The listing builds one solid part. Answer for the finished solid, in the listing's coordinates (mm). Face numbers are marked on the shaded views. A direction names the side the tool comes from. Give positions to 0.01 mm unless a question says otherwise; leave off trailing zeros. Order: outer loops, then holes, each group sorted by start corner. A loop starts at its lowest first (then second) coordinate and runs counter-clockwise, first axis right, second up. Notation, with made-up numbers: (34.25, 56) - (68.25, 56) arc R18 cw to (68.25, 87) - close; hole circle Ø8 at (-5, 69). An arc over 180 degrees is marked (long way). Answer as a JSON object with one key per item and string values. Group by question number.
Q1. A cutting plane is placed at B-B, the plane y = -4.5. Give the vertices of the cut face in (x, z), and give its area (3 significant figures).
Q2. A cutting plane is placed at D-D, the plane y = -26. Give the vertices of the cut face in (x, z).
Q3. A cutting plane is placed at C-C, the plane x = 9.7. Give the vertices of the cut face in (y, z), and give its area (3 significant figures).
Q4. For the marked faces 4, 5, 6, 7 and 8, determine the directions among +Z, -Z, +X, -X, +Y, -Y from which every point of the face is accessible in a straight line to the end or side of a thin tool.
Q5. Consider line 1 (Z direction, x = 9.7, y = -10.35); line 2 (Y direction, x = -21, z = -1.25); line 3 (X direction, y = -25, z = 4.25). Determine where each line is inside the solid, lowest interval first.
Q6. The mould has two halves that part along Y. Classify the marked faces 1, 2 and 3: released by +Y, released by -Y, zero draft, split by the parting line, or undercut.
Q7. A cutting plane is placed at A-A, the plane x = -25.2. Give the vertices of the cut face in (y, z).
Q8. Given pin 1 (4 mm diameter, centred on x = -6.5, z = -2, fed in from +Y); pin 2 (4 mm diameter, centred on y = -21, z = 4.5, fed in from -X); pin 3 (6.5 mm diameter, centred on y = -7.5, z = 1.5, fed in from +X), each flat-ended and moving along its own axis, determine where each tip first touches the part or whether it passes through.
from build123d import *

# Parameters (mm, degrees)
BOSS_EXTRU_1_DEPTH            = 6.5
BOSS_EXTRU_1_DEPTH_BACK       = 6.5
ENL_V_MAT_EXTRU_1_DEPTH       = 2.8
ESQUISSE3_R                   = 6
BOSS_EXTRU_2_DEPTH            = 3.9
BOSS_EXTRU_3_DEPTH            = 3.8
BOSS_EXTRU_4_DEPTH            = 2
DIAM_TRE_DU_PER_AGE_4_0_4_1_D = 4
DIAM_TRE_DU_PER_AGE_4_0_4_2_D = 4
ESQUISSE10_W                  = 7
ESQUISSE10_H                  = 5
BOSS_EXTRU_5_DEPTH            = 7
D_POUILLE1_ANGLE              = 5
ESQUISSE11_W                  = 2
ESQUISSE11_H                  = 2.5
ENL_V_MAT_EXTRU_2_DEPTH       = 22.8
ENL_V_MAT_EXTRU_3_REACH       = 23.8
ESQUISSE12_W                  = 2
ESQUISSE12_H                  = 2.5


with BuildPart() as part:
    # Esquisse1 → Boss.-Extru.1 (new body, two sides)
    with BuildSketch(Plane.XY) as boss_extru_1_sk:
        Polygon((-22.5, -11.2), (-22.5, -31.2), (7, -31.2), (7, -11.2), (12, -11.2), (12, -9.4), (7, -9.4), (7, -3.7), (-22.5, -3.7), (-22.5, -9.4), (-27.5, -9.4), (-27.5, -11.2), align=None)
    extrude(amount=BOSS_EXTRU_1_DEPTH)
    extrude(boss_extru_1_sk.sketch, amount=-BOSS_EXTRU_1_DEPTH_BACK)

    # Esquisse2 → Enl_v. mat.-Extru.1 (cut)
    with BuildSketch(Plane(origin=(0, -3.7, 0), x_dir=(1, 0, 0), z_dir=(0, 1, 0))):
        Polygon((-5.5, 6.5), (-5.5, 5.5), (-21.1, 5.5), (-21.1, -5.5), (-5.5, -5.5), (-5.5, -6.5), (-22.5, -6.5), (-22.5, 6.5), align=None)
    extrude(amount=-ENL_V_MAT_EXTRU_1_DEPTH, mode=Mode.SUBTRACT)

    # Esquisse3 → Boss.-Extru.2 (add)
    with BuildSketch(Plane(origin=(0, -3.7, 0), x_dir=(1, 0, 0), z_dir=(0, 1, 0))):
        Circle(ESQUISSE3_R)
    extrude(amount=BOSS_EXTRU_2_DEPTH)

    # Esquisse4 → Boss.-Extru.3 (add)
    with BuildSketch(Plane(origin=(0, 0.2, 0), x_dir=(1, 0, 0), z_dir=(0, 1, 0))):
        Polygon((0.332133069, 2.629103958), (0, 3), (-0.332133069, 2.629103958), (-0.746069661, 2.905749483), (-0.975530065, 2.463907688), (-1.445261022, 2.62892004), (-1.557630919, 2.143895035), (-2.053641318, 2.186905882), (-2.041860093, 1.689173573), (-2.532983777, 1.607480385), (-2.397791689, 1.128315123), (-2.853169549, 0.927050983), (-2.603061214, 0.496560484), (-2.994080185, 0.188371559), (-2.64477083, -0.166394877), (-2.946861752, -0.562143944), (-2.520299768, -0.818895035), (-2.714481157, -1.277337875), (-2.237469003, -1.419941007), (-2.311539728, -1.912271969), (-1.814049831, -1.931766863), (-1.763355757, -2.427050983), (-1.276647236, -2.322212702), (-1.104373658, -2.789329458), (-0.659028201, -2.566745377), (-0.375999701, -2.976344104), (0, -2.65), (0.375999701, -2.976344104), (0.659028201, -2.566745377), (1.104373658, -2.789329458), (1.276647236, -2.322212702), (1.763355757, -2.427050983), (1.814049831, -1.931766863), (2.311539728, -1.912271969), (2.237469003, -1.419941007), (2.714481157, -1.277337875), (2.520299768, -0.818895035), (2.946861752, -0.562143944), (2.64477083, -0.166394877), (2.994080185, 0.188371559), (2.603061214, 0.496560484), (2.853169549, 0.927050983), (2.397791689, 1.128315123), (2.532983777, 1.607480385), (2.041860093, 1.689173573), (2.053641318, 2.186905882), (1.557630919, 2.143895035), (1.445261022, 2.62892004), (0.975530065, 2.463907688), (0.746069661, 2.905749483), align=None)
    extrude(amount=BOSS_EXTRU_3_DEPTH)

    # Esquisse5 → Boss.-Extru.4 (add)
    with BuildSketch(Plane(origin=(0, -3.7, 0), x_dir=(1, 0, 0), z_dir=(0, 1, 0))):
        with BuildLine():
            Line((-9.848350116, 4.9), (0, 4.9))
            Line((0, 4.9), (0, -4.9))
            Line((0, -4.9), (-9.848350116, -4.9))
            ThreePointArc((-9.848350116, -4.9), (-11, 0), (-9.848350116, 4.9))
        make_face()
    extrude(amount=BOSS_EXTRU_4_DEPTH)

    # Diam_tre du per_age _4.0 _4_1 (through all)
    with Locations(Plane(origin=(0, -9.4, 0), x_dir=(1, 0, 0), z_dir=(0, 1, 0))):
        with Locations((-25.2, 0)):
            Hole(DIAM_TRE_DU_PER_AGE_4_0_4_1_D / 2)

    # Diam_tre du per_age _4.0 _4_2 (through all)
    with Locations(Plane(origin=(0, -9.4, 0), x_dir=(1, 0, 0), z_dir=(0, 1, 0))):
        with Locations((9.7, 0)):
            Hole(DIAM_TRE_DU_PER_AGE_4_0_4_2_D / 2)

    # Esquisse10 → Boss.-Extru.5 (add)
    with BuildSketch(Plane(origin=(7, 0, 0), x_dir=(0, 0, -1), z_dir=(1, 0, 0))):
        with Locations((0, -24.7)):
            Rectangle(ESQUISSE10_W, ESQUISSE10_H)
    extrude(amount=BOSS_EXTRU_5_DEPTH)

    # D_pouille1
    d_pouille1_faces = [part.faces().sort_by_distance(p)[0] for p in [
        (10.5, -27.2, 0),
        (10.5, -24.7, -3.5),
        (10.5, -22.2, 0),
        (10.5, -24.7, 3.5),
    ]]
    draft(d_pouille1_faces, Plane(origin=(7, -11.2, -6.5), x_dir=(0, 1, 0), z_dir=(1, 0, 0)), D_POUILLE1_ANGLE)

    # Esquisse11 → Enl_v. mat.-Extru.2 (cut, through all)
    with BuildSketch(Plane(origin=(0, -9.4, 0), x_dir=(1, 0, 0), z_dir=(0, 1, 0))):
        with Locations((-26.5, 0)):
            Rectangle(ESQUISSE11_W, ESQUISSE11_H)
    extrude(amount=-ENL_V_MAT_EXTRU_2_DEPTH, mode=Mode.SUBTRACT)

    # Esquisse12 → Enl_v. mat.-Extru.3 (cut, up to next)
    with BuildSketch(Plane(origin=(0, -9.4, 0), x_dir=(1, 0, 0), z_dir=(0, 1, 0)), mode=Mode.PRIVATE) as enl_v_mat_extru_3_sk1:
        with Locations((11, 0)):
            Rectangle(ESQUISSE12_W, ESQUISSE12_H)
    enl_v_mat_extru_3_tool1 = extrude(enl_v_mat_extru_3_sk1.sketch, amount=-ENL_V_MAT_EXTRU_3_REACH, mode=Mode.PRIVATE) & part.part
    add(enl_v_mat_extru_3_tool1.solids().sort_by_distance((11, -9.4, 0))[0], mode=Mode.SUBTRACT)


solid = part.part
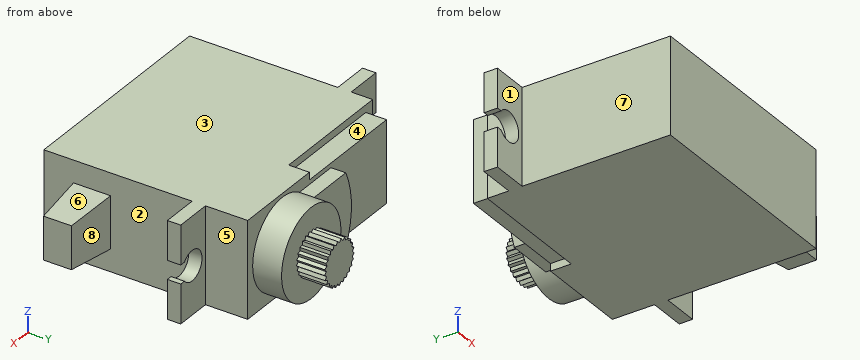
Reply:
{
 "1": {"outline": "(-21.1, -5.5) - (-5.5, -5.5) - (-5.5, -6.5) - (7, -6.5) - (7, 6.5) - (-5.5, 6.5) - (-5.5, 5.5) - (-21.1, 5.5) - close", "area": "334 mm^2"},
 "2": {"outline": "(-22.5, -6.5) - (7, -6.5) - (7, -3.5) - (14, -2.89) - (14, 2.89) - (7, 3.5) - (7, 6.5) - (-22.5, 6.5) - close"},
 "3": {"outline": "(-26.96, -3.26) - (-22.44, -3.26) - (-22.44, 3.26) - (-26.96, 3.26) - close; (-11.2, -6.5) - (-9.4, -6.5) - (-9.4, -2) - (-11.2, -2) - close; (-11.2, 2) - (-9.4, 2) - (-9.4, 6.5) - (-11.2, 6.5) - close", "area": "45.8 mm^2"},
 "4": {"face 4": "+Z, -X, +Y", "face 5": "+Z, -Z, +X, +Y", "face 6": "+Z, +X, -Y", "face 7": "+Z, -Z, -X, -Y", "face 8": "+Z, -Z, +X"},
 "5": {"line 1": "z = -6.5 to -2, 2 to 6.5", "line 2": "y = -31.2 to -3.7", "line 3": "x = -22.5 to 7"},
 "6": {"face 1": "released by -Y", "face 2": "undercut", "face 3": "zero draft"},
 "7": {"outline": "(-11.2, -6.5) - (-9.4, -6.5) - (-9.4, -2) - (-11.2, -2) - close; (-11.2, 2) - (-9.4, 2) - (-9.4, 6.5) - (-11.2, 6.5) - close"},
 "8": {"pin 1": "stops at y = 0.2", "pin 2": "stops at x = -22.5", "pin 3": "stops at x = 12"}
}
